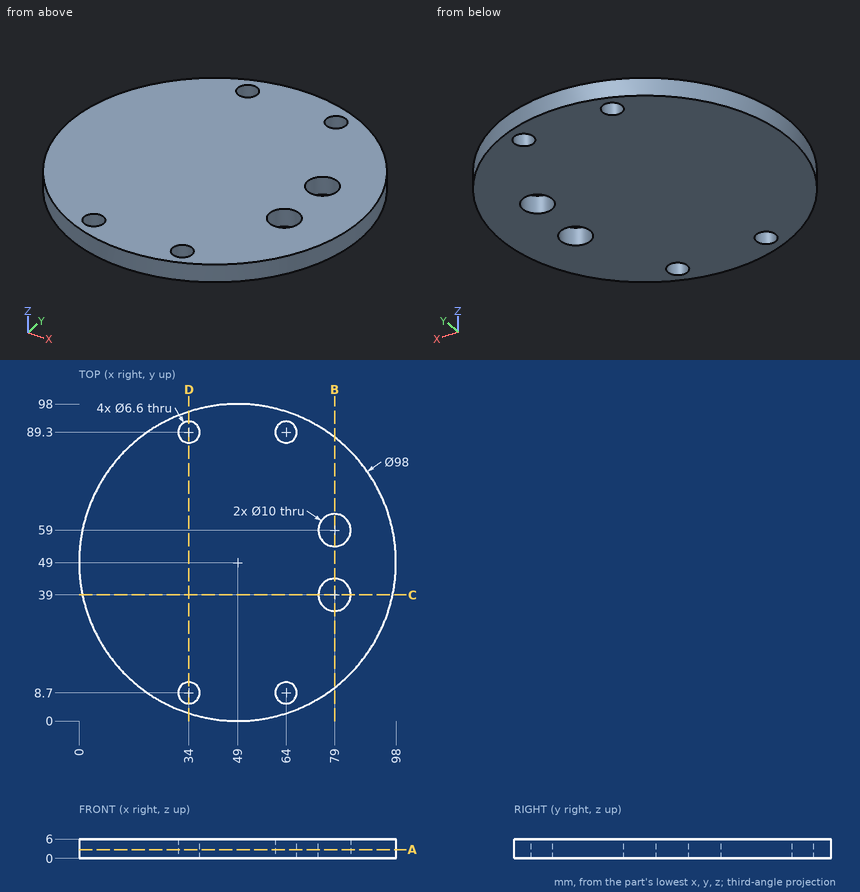
The figure shows three views and two pictorial views of one solid part (mm, origin at its lowest corner). Answer the questions. Coordinates: 2 decimals unless noted, no trailing zeros. Write each loop counter-clockwise with the first axis right and the second up, starting at its lowest first coordinate (ties: lowest second). Pieces come first, ordered by that corner, then holes.
1. The part is cut by section A-A, the plane z = 2.7. Write down the section's boundary in (x, y).
Results list:
outline: circle Ø98 at (49, 49); hole circle Ø6.6 at (34, 8.7); hole circle Ø6.6 at (34, 89.3); hole circle Ø6.6 at (64, 8.7); hole circle Ø6.6 at (64, 89.3); hole circle Ø10 at (79, 39); hole circle Ø10 at (79, 59)
2. The part is cut by section D-D, the plane x = 34. Write down the section's boundary in (y, z), and give its area (3 significant figures).
Results list:
outline: (2.35, 0) - (5.4, 0) - (5.4, 6) - (2.35, 6) - close; (12, 0) - (86, 0) - (86, 6) - (12, 6) - close; (92.6, 0) - (95.65, 0) - (95.65, 6) - (92.6, 6) - close
area: 481 mm2
3. The part is cut by section C-C, the plane y = 39. Write down the section's boundary in (x, z).
Results list:
outline: (1.03, 0) - (74, 0) - (74, 6) - (1.03, 6) - close; (84, 0) - (96.97, 0) - (96.97, 6) - (84, 6) - close
4. Flat-ended cylindrical pins translate along their axes: pin 1 (11.5 mm diameter, centred on x = 79, y = 59, fed in from +Z); pin 2 (6 mm diameter, centred on x = 34, y = 89.3, fed in from +Z). Find the tip coordinate at first contact, or state that the pin passes through.
Results list:
pin 1: stops at z = 6
pin 2: passes through
5. Consider line 1 along Y through (x, z) = (79, 3.05); line 2 along Y through (x, z) = (79.5, 1.7); line 3 along X through (y, z) = (89, 1.9). Determine where each line is inside the solid, lowest interval first.
Results list:
line 1: y = 10.26 to 34, 44 to 54, 64 to 87.74
line 2: y = 10.65 to 34.03, 43.97 to 54.03, 63.97 to 87.35
line 3: x = 20.7 to 30.71, 37.29 to 60.71, 67.29 to 77.3
6. The part is cut by section B-B, the plane x = 79. Write down the section's boundary in (y, z), and give its area (3 significant figures).
Results list:
outline: (10.26, 0) - (34, 0) - (34, 6) - (10.26, 6) - close; (44, 0) - (54, 0) - (54, 6) - (44, 6) - close; (64, 0) - (87.74, 0) - (87.74, 6) - (64, 6) - close
area: 345 mm2
